```python
from build123d import *
from build123d.topology import SkipClean

# Parameters (mm, degrees)
SKETCH1_R           = 49.5046
BOSS_EXTRUDE1_DEPTH = 5.08
SKETCH2_R           = 47.625
BOSS_EXTRUDE2_DEPTH = 3.175
SKETCH3_R           = 3.96875
SKETCH3_R_2         = 6.35
CUT_EXTRUDE1_DEPTH  = 71.495076901
CUT_EXTRUDE2_DEPTH  = 71.194139658
SKETCH5_R           = 54.412278645
CUT_EXTRUDE3_DEPTH  = 3.175
SKETCH6_R           = 1.5875
CUT_EXTRUDE4_DEPTH  = 71.194139658
SKETCH7_R           = 3.175
CUT_EXTRUDE5_DEPTH  = 71.194139658


with BuildPart() as part:
    # Sketch1 → Boss-Extrude1 (new body)
    with BuildSketch(Plane.XY):
        Circle(SKETCH1_R)
    extrude(amount=BOSS_EXTRUDE1_DEPTH)

    # Sketch2 → Boss-Extrude2 (add)
    with BuildSketch(Plane.XY.offset(5.08)):
        Circle(SKETCH2_R)
    extrude(amount=BOSS_EXTRUDE2_DEPTH)

    # Sketch3 → Cut-Extrude1 (cut, through all)
    with BuildSketch(Plane.XY.offset(8.255)):
        with Locations((-31.75, 0)):
            Circle(SKETCH3_R)
        with Locations((31.75, 0)):
            Circle(SKETCH3_R)
        with Locations((-12.7, -31.166793627)):
            Circle(SKETCH3_R_2)
        with Locations((12.7, -31.166793627)):
            Circle(SKETCH3_R_2)
    extrude(amount=-CUT_EXTRUDE1_DEPTH, mode=Mode.SUBTRACT)

    # Sketch4 → Cut-Extrude2 (cut, through all)
    with SkipClean():  # the faces are left unmerged after this step: merging them gives an invalid solid
        with BuildSketch(Plane.XY.offset(5.08)):
            with BuildLine():
                Line((-50.165, 0), (-47.625, 0))
                ThreePointArc((-47.625, 0), (0, -47.625), (47.625, 0))
                Line((47.625, 0), (50.165, 0))
                ThreePointArc((50.165, 0), (0, -50.165), (-50.165, 0))
            make_face()
        extrude(amount=-CUT_EXTRUDE2_DEPTH, mode=Mode.SUBTRACT)

    # Sketch5 → Cut-Extrude3 (cut)
    with BuildSketch(Plane.XY.offset(8.255)):
        Circle(SKETCH5_R)
    extrude(amount=-CUT_EXTRUDE3_DEPTH, mode=Mode.SUBTRACT)

    # Sketch6 → Cut-Extrude4 (cut, through all)
    with BuildSketch(Plane(origin=(0, 0, 0), x_dir=(-1, 0, 0), z_dir=(0, 0, -1))):
        with Locations((-47.625, -1.5875)):
            Circle(SKETCH6_R)
        with Locations((47.625, -1.5875)):
            Circle(SKETCH6_R)
    extrude(amount=-CUT_EXTRUDE4_DEPTH, mode=Mode.SUBTRACT)

    # Sketch7 → Cut-Extrude5 (cut, through all)
    with BuildSketch(Plane.XY.offset(5.08)):
        with Locations((0, -34.925)):
            Circle(SKETCH7_R)
    extrude(amount=-CUT_EXTRUDE5_DEPTH, mode=Mode.SUBTRACT)


solid = part.part
```
The listing builds one solid part. Answer for the finished solid, in the listing's coordinates (mm). Give positions to 0.01 mm unless a question says otherwise; leave off trailing zeros. Order: outer loops, then holes, each group sorted by start corner. A loop starts at its lowest first (then second) coordinate and runs counter-clockwise, first axis right, second up. Notation, with made-up numbers: (84.25, -13) -> (133.25, -13) arc R37 cw to (133.25, 25) -> close; hole circle Ø8 at (-35.75, 50). An arc over 180 degrees is marked (long way). Answer as a JSON object with one key per item and string values. Group by question number.
Item 1: The part is cut by section C-C on x = -16. Write down the section's boundary in (y, z).
Item 2: The part is cut by section D-D on y = 15. Write down the section's boundary in (x, z).
Item 3: The part is cut by section A-A on x = 0. Write down the section's boundary in (y, z) (3 decimals).
Item 4: The part is cut by section B-B on z = 4.15. Give the number of separate pieces and of enclosed holes in the cut face, and give its area (3 significant figures).
Item 5: Flat-ended cylindrical pins translate along their axes: pin 1 (1.5 mm diameter, centred on x = 48.5, z = 3, fed in from -Y); pin 2 (10.5 mm diameter, centred on x = 31.75, y = 0, fed in from -Z); pin 3 (1.5 mm diameter, centred on x = -14.5, z = 3.5, fed in from -Y); pin 4 (3 mm diameter, centred on x = 30, z = 2, fed in from +Y). Find the tip coordinate at first contact, or state that the pin passes through.
Item 6: Consider L1, parallel to X at y = -34.5, z = 3.65; L2, parallel to Y at x = 0, z = 1.8 (3 decimals); L3, parallel to Y at x = 17.5, z = 4.4. Determine where each line is inside the solid, lowest interval first. Write a range as from..to.
Item 7: Determine the mould class of faces 1 (the cylindrical face through (-0.688, -38.024, 2.576)), 2 (the cylindrical face through (-46.04, -1.5, 2.5)), 3 (the flat face through (-1, 2, 0)) for opening direction X: pulls with the +X half, pulls with the -X half, needs draft (parallel to the pull), parting line crosses it, or undercut.
Result set:
{
 "1": {"outline": "(-44.86, 0) -> (-36.59, 0) -> (-36.59, 5.08) -> (-44.86, 5.08) -> close; (-25.74, 0) -> (46.85, 0) -> (46.85, 5.08) -> (-25.74, 5.08) -> close"},
 "2": {"outline": "(-47.18, 0) -> (47.18, 0) -> (47.18, 5.08) -> (-47.18, 5.08) -> close"},
 "3": {"outline": "(-47.625, 0) -> (-38.1, 0) -> (-38.1, 5.08) -> (-47.625, 5.08) -> close; (-31.75, 0) -> (49.505, 0) -> (49.505, 5.08) -> (-31.75, 5.08) -> close"},
 "4": {"separate pieces": "1", "enclosed holes": "5", "area": "7,020 mm²"},
 "5": {"pin 1": "y = 0", "pin 2": "z = 0", "pin 3": "y = -45.6", "pin 4": "y = 40.48"},
 "6": {"L1": "-32.83..-18.1, -7.3..-3.15, 3.15..7.3, 18.1..32.83", "L2": "-47.625..-38.1, -31.75..49.505", "L3": "-44.29..-35.32, -27.01..46.31"},
 "7": {"face 1": "undercut", "face 2": "pulls with the -X half", "face 3": "needs draft"}
}
